Can you work these out from the drawing? Everything is in mm from the part's minimum corner. Give positions to 0.01 mm unless a question says otherwise; leave off trailing zeros. Order: outer loops, then holes, each group sorted by start corner. A loop starts at its lowest first (then second) coordinate and runs counter-clockwise, first axis right, second up. Notation, with made-up numbers: (-15.5, 15.5) - (14.5, 15.5) arc R20 ccw to (14.5, 48.5) - close; hole circle Ø10 at (-22, 80.5). An arc over 180 degrees is marked (long way). One line per question, with ' | ' between items.
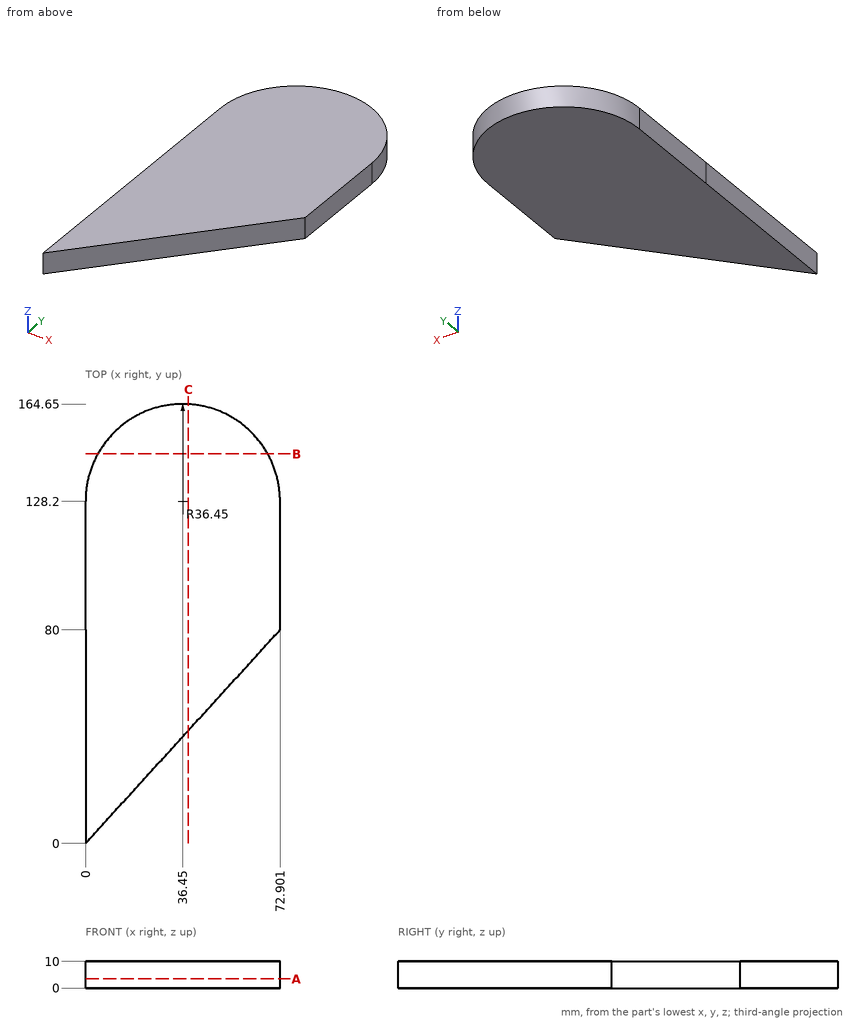
(1) If I drill on line 1 (X direction, y = 11, z = 5) (1 decimal); line 2 (Y direction, x = 43, z = 5) (1 decimal); line 3 (Y direction, x = 15, z = 9.75), over which ranges is the centre line in solid material (lowest first)?
Answer below:
line 1: 0 to 10 | line 2: 47.2 to 164.1 | line 3: 16.46 to 157.67
(2) Imagine slicing it at C-C (x = 38.5). List the corners of the cut face in (y, z) for me, and give its area (3 significant figures).
Answer below:
outline: (42.25, 0) - (164.59, 0) - (164.59, 10) - (42.25, 10) - close | area: 1,220 mm^2
(3) Imagine slicing it at A-A (z = 3.5). List the corners of the cut face in (x, y) for me, and give its area (3 significant figures).
Answer below:
outline: (0, 0) - (72.9, 80) - (72.9, 128.2) arc R36.45 ccw to (0, 128.2) - close | area: 8,520 mm^2
(4) Will these pins go through, and if not, where does the flat tip stop? pin 1 (1 mm diameter, centred on y = 142, z = 6, fed in from -X); pin 2 (4 mm diameter, centred on x = 48, z = 6, fed in from +Y).
Answer below:
pin 1: x = 2.51 | pin 2: y = 163.38
(5) Imagine slicing it at B-B (y = 146). List the corners of the cut face in (x, z) for me.
Answer below:
outline: (4.64, 0) - (68.26, 0) - (68.26, 10) - (4.64, 10) - close
